Geometry check sheet. Reference: the model listing, model coordinates, mm. A direction names the side the tool comes from. Round coordinates to 2 decimals unless told otherwise and drop trailing zeros. Order: outer loops, then holes, each group sorted by start corner. A loop starts at its lowest first (then second) coordinate and runs counter-clockwise, first axis right, second up. Notation, with made-up numbers: (35.5, 11.25) -> (49.5, 11.25) arc R18 cw to (49.5, 21.25) -> close; hole circle Ø6 at (19.25, 10.5). An arc over 180 degrees is marked (long way). Use a Markdown table: item, result. Add a question column.
Item 1: Sectioned sample at A-A, the plane z = -4.25. Record the cut outline in (x, y).
Item 2: Set-up check for faces 3 (the cylindrical face through (40.759, -0.28, -4.015)), 4 (the cylindrical face through (28.801, 15.437, 3.035)), 5 (the cylindrical face through (28.215, 10.301, 4.637)), 6 (the flat face through (28.5, -15, 5)), 7 (the flat face through (18, 0, 2.75)): record each of +Z, -Z, +X, -X, +Y, -Y from which the full face is reachable in a straight line by a thin tool's end or side.
Item 3: Gauge pin test, flat ends, axial feed: pin 1 Ø1.4 at (y, z) = (-13.5, 4.5) entering from +X; pin 2 Ø0.5 at (y, z) = (-15.5, 5) entering from -X; pin 3 Ø19 at (x, y) = (17, -5) entering from -Z; pin 4 Ø1.5 at (x, y) = (26, 15.5) entering from -Z. Record the tip position at first contact, or that the pin passes through.
Item 4: Material ranges on probe 1 along X at (y, z) = (-11, 0.25); probe 2 along Z at (x, y) = (37, 8.5); probe 3 along X at (y, z) = (11.5, 0.75), recorded low to high. Write a range as [from, to].
Item 5: Mould release check, pull along X, two halves, no side actions. Record for faces 1 (the flat face through (1, 20, 3)), 2 (the cylindrical face through (28.199, -10.285, 4.637)): pulls with the +X half, pulls with the -X half, needs draft (parallel to the pull), parting line crosses it, or undercut.
Item 6: Sectioned sample at B-B, the plane x = 23. Record the cut outline in (y, z).
from build123d import *

# Parameters (mm, degrees)
F0_R          = 2.75
F1_DEPTH      = 20
F1_DEPTH_BACK = 20
F2_W          = 20
F2_H          = 10
F3_DEPTH      = 2.75
F4_R          = 1


with BuildPart() as f1:
    # F0 (on Front) → F1 (new body, two sides)
    with BuildSketch(Plane.XZ) as f1_sk:
        with BuildLine():
            Line((37, 5.5), (0, 5.5))
            ThreePointArc((0, 5.5), (-3.8890872965, -3.8890872965), (5.5, 0))
            Line((5.5, 0), (5.5, 1.75))
            ThreePointArc((5.5, 1.75), (5.7928932188, 2.4571067812), (6.5, 2.75))
            Line((6.5, 2.75), (30.5, 2.75))
            ThreePointArc((30.5, 2.75), (31.2071067812, 2.4571067812), (31.5, 1.75))
            Line((31.5, 1.75), (31.5, 0))
            ThreePointArc((31.5, 0), (40.8890872965, -3.8890872965), (37, 5.5))
        make_face()
        Circle(F0_R, mode=Mode.SUBTRACT)
        with Locations((37, 0)):
            Circle(F0_R, mode=Mode.SUBTRACT)
    extrude(amount=F1_DEPTH)
    extrude(f1_sk.sketch, amount=-F1_DEPTH_BACK)

    # F2 (on face) → F3 (cut, through all)
    with BuildSketch(Plane(origin=(0, 0, 2.75), x_dir=(1, 0, 0), z_dir=(0, 0, -1))):
        with Locations((18.5, -15)):
            Rectangle(F2_W, F2_H)
        with Locations((18.5, 15)):
            Rectangle(F2_W, F2_H)
    extrude(amount=-F3_DEPTH, mode=Mode.SUBTRACT)

    # F4
    f4_edges = [f1.edges().sort_by_distance(p)[0] for p in [
        (8.5, -15, 2.75),
        (8.5, 15, 2.75),
        (28.5, 15, 2.75),
        (28.5, -15, 2.75),
        (8.5, -10, 4.125),
        (28.5, -10, 4.125),
        (28.5, 10, 4.125),
        (8.5, 10, 4.125),
        (18.5, 10, 2.75),
        (18.5, -10, 2.75),
    ]]
    fillet(f4_edges, radius=F4_R)


solid = f1.part
Found:
| question | item | result |
|---|---|---|
| 1 | outline | (-3.49, -20) -> (3.49, -20) -> (3.49, 20) -> (-3.49, 20) -> close; (33.51, -20) -> (40.49, -20) -> (40.49, 20) -> (33.51, 20) -> close |
| 2 | face 3 | +Y, -Y |
| 2 | face 4 | -Z, +Y |
| 2 | face 5 | +Z, -Z, +Y |
| 2 | face 6 | +Z, -Z, -Y |
| 2 | face 7 | -Z, +Y, -Y |
| 3 | pin 1 | stops at x = 40.98 |
| 3 | pin 2 | stops at x = -2.77 |
| 3 | pin 3 | stops at z = 2.75 |
| 3 | pin 4 | passes through |
| 4 | probe 1 | x = [-5.49, -2.74], [2.74, 5.5], [31.5, 34.26], [39.74, 42.49] |
| 4 | probe 2 | z = [-5.5, -2.75], [2.75, 5.5] |
| 4 | probe 3 | x = [-5.45, -2.65], [2.65, 5.5], [31.5, 34.35], [39.65, 42.45] |
| 5 | face 1 | needs draft |
| 5 | face 2 | undercut |
| 6 | outline | (-10, 3.75) arc R1 ccw to (-9, 2.75) -> (9, 2.75) arc R1 ccw to (10, 3.75) -> (10, 5.5) -> (-10, 5.5) -> close |
